Could you check a few things on this model? Use its own coordinates, in mm. A direction names the side the tool comes from. Coordinates: 2 decimals unless noted, no trailing zeros. One line per question, with ' | ' between items.
from build123d import *

# Parameters (mm, degrees)
SKETCH1_R           = 7.62
BOSS_EXTRUDE1_DEPTH = 38.1
SKETCH5_R           = 6.096
SKETCH3_R           = 6.450000054
SKETCH6_R           = 10.218046867
SKETCH6_R_2         = 7.62
BOSS_EXTRUDE2_DEPTH = 14.0199999
CHAMFER1_SIZE       = 2.54


with BuildPart() as part:
    # Sketch1 → Boss-Extrude1 (new body)
    with BuildSketch(Plane(origin=(0, 0, 0), x_dir=(1, 0, 0), z_dir=(0, 1, 0))):
        with Locations(Location((0, 0, 0), (0, 0, 90))):
            Circle(SKETCH1_R)
    extrude(amount=BOSS_EXTRUDE1_DEPTH)

    # Sketch4 → Motor Shaft Couple section 0
    with BuildSketch(Plane(origin=(0, 19.0999999, 0), x_dir=(1, 0, 0), z_dir=(0, 1, 0))):
        with BuildLine():
            Line((-2.569046516, 2.8), (2.569046516, 2.8))
            ThreePointArc((2.569046516, 2.8), (0, -3.8), (-2.569046516, 2.8))
        make_face()
    # Sketch2 → Motor Shaft Couple section 1
    with BuildSketch(Plane(origin=(0, 38.1, 0), x_dir=(1, 0, 0), z_dir=(0, 1, 0))):
        with BuildLine():
            Line((-2.720293955, 3.1999996), (2.720293955, 3.1999996))
            ThreePointArc((2.720293955, 3.1999996), (0, -4.1999996), (-2.720293955, 3.1999996))
        make_face()
    loft(mode=Mode.SUBTRACT)

    # Sketch5 → Dowel Couple section 0
    with BuildSketch(Plane(origin=(0, 14.0199999, 0), x_dir=(1, 0, 0), z_dir=(0, 1, 0))):
        Circle(SKETCH5_R)
    # Sketch3 → Dowel Couple section 1
    with BuildSketch(Plane.XZ):
        Circle(SKETCH3_R)
    loft(mode=Mode.SUBTRACT)

    # Sketch6 → Boss-Extrude2 (add)
    with BuildSketch(Plane.XZ):
        with Locations(Location((0, 0, 0), (0, 0, 270))):
            Circle(SKETCH6_R)
        with Locations(Location((0, 0, 0), (0, 0, 270))):
            Circle(SKETCH6_R_2, mode=Mode.SUBTRACT)
    extrude(amount=-BOSS_EXTRUDE2_DEPTH)

    # Chamfer1
    chamfer1_edges = [part.edges().sort_by_distance(p)[0] for p in [
        (0, 14.0199999, 7.62),
    ]]
    chamfer(chamfer1_edges, length=CHAMFER1_SIZE)


solid = part.part
1) I need wall thicknesses on line 1 along Y through (x, z) = (-1.75, -5.5); line 2 along X through (y, z) = (23.5, -2.75); line 3 along X through (y, z) = (21, -2.5). Which ranges of each line are inside material? Lowest first, please. Write a range as from..to.
Data:
line 1: 14.02..38.1 | line 2: -7.11..-2.75, 2.75..7.11 | line 3: -7.2..-2.91, 2.91..7.2
2) On a 3-axis mill with a long thin cutter (end or side, diameter ignored), from which of +Z, -Z, +X, -X, +Y, -Y can I reach the whole of each face in a straight line? I mean faces 4 (the face through (5.986, 6.912, -1.885)), 5 (the face through (0, 19.1, 0)), 6 (the face through (-9.975, 6.912, 2.215)). Say none if no direction works.
Data:
face 4: -Y | face 5: +Y | face 6: +Y, -Y
3) I'm going to push flat-ended pins straight in: pin 1 Ø5 at (x, y) = (5, 11) entering from +Z; pin 2 Ø1.5 at (x, z) = (2.5, 1.5) entering from +Y; pin 3 Ø1 at (x, z) = (5.5, -0.5) entering from -Y. Where does each tip first touch, or does it pass through?
Data:
pin 1: z = 9.91 | pin 2: y = 19.1 | pin 3: y = 14.02
4) We'd pull the mould along X, two halves only. Please class faces 1 (the face through (3.3, 38.1, -3.3)), 2 (the face through (0, 14.02, 0)), 3 (the face through (-7.555, 27.179, 0.992)): pulls with the +X half, pulls with the -X half, needs draft (parallel to the pull), parting line crosses it, or undercut.
Data:
face 1: needs draft | face 2: undercut | face 3: parting line crosses it
